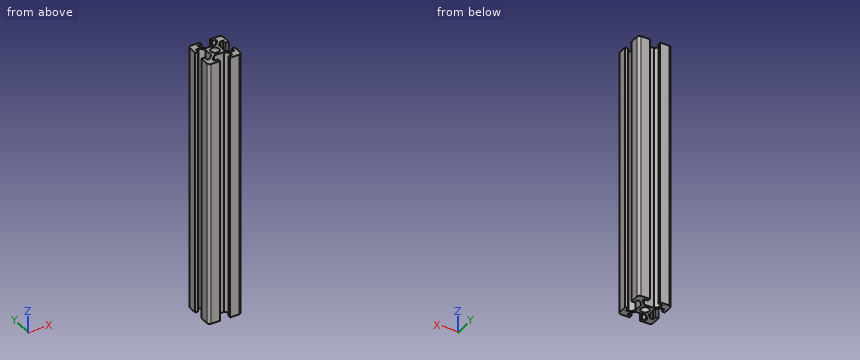
from build123d import *

# Parameters (mm, degrees)
SKETCH_1_R      = 2.5
EXTRUDE_2_DEPTH = 160
SCALE1_SCALE    = 2.5


with BuildPart() as part:
    # 草图1 → 凸台-拉伸2 (new body)
    with BuildSketch(Plane.XY):
        with BuildLine():
            Line((5.5, -8.2), (5.5, -6.560660172))
            Line((5.5, -6.560660172), (2.939339828, -4))
            Line((2.939339828, -4), (-2.939339828, -4))
            Line((-2.939339828, -4), (-5.5, -6.560660172))
            Line((-5.5, -6.560660172), (-5.5, -8.2))
            Line((-5.5, -8.2), (-3.1, -8.2))
            Line((-3.1, -8.2), (-3.1, -10))
            Line((-3.1, -10), (-8.5, -10))
            ThreePointArc((-8.5, -10), (-9.560660172, -9.560660172), (-10, -8.5))
            Line((-10, -8.5), (-10, -3.1))
            Line((-10, -3.1), (-8.2, -3.1))
            Line((-8.2, -3.1), (-8.2, -5.5))
            Line((-8.2, -5.5), (-6.560660172, -5.5))
            Line((-6.560660172, -5.5), (-4, -2.939339828))
            Line((-4, -2.939339828), (-4, 2.939339828))
            Line((-4, 2.939339828), (-6.560660172, 5.5))
            Line((-6.560660172, 5.5), (-8.2, 5.5))
            Line((-8.2, 5.5), (-8.2, 3.1))
            Line((-8.2, 3.1), (-10, 3.1))
            Line((-10, 3.1), (-10, 8.5))
            ThreePointArc((-10, 8.5), (-9.560660172, 9.560660172), (-8.5, 10))
            Line((-8.5, 10), (-3.1, 10))
            Line((-3.1, 10), (-3.1, 8.2))
            Line((-3.1, 8.2), (-5.5, 8.2))
            Line((-5.5, 8.2), (-5.5, 6.560660172))
            Line((-5.5, 6.560660172), (-2.939339828, 4))
            Line((-2.939339828, 4), (2.939339828, 4))
            Line((2.939339828, 4), (5.5, 6.560660172))
            Line((5.5, 6.560660172), (5.5, 8.2))
            Line((5.5, 8.2), (3.1, 8.2))
            Line((3.1, 8.2), (3.1, 10))
            Line((3.1, 10), (8.5, 10))
            ThreePointArc((8.5, 10), (9.560660172, 9.560660172), (10, 8.5))
            Line((10, 8.5), (10, 3.1))
            Line((10, 3.1), (8.2, 3.1))
            Line((8.2, 3.1), (8.2, 5.5))
            Line((8.2, 5.5), (6.560660172, 5.5))
            Line((6.560660172, 5.5), (4, 2.939339828))
            Line((4, 2.939339828), (4, -2.939339828))
            Line((4, -2.939339828), (6.560660172, -5.5))
            Line((6.560660172, -5.5), (8.2, -5.5))
            Line((8.2, -5.5), (8.2, -3.1))
            Line((8.2, -3.1), (10, -3.1))
            Line((10, -3.1), (10, -8.5))
            ThreePointArc((10, -8.5), (9.560660172, -9.560660172), (8.5, -10))
            Line((8.5, -10), (3.1, -10))
            Line((3.1, -10), (3.1, -8.2))
            Line((3.1, -8.2), (5.5, -8.2))
        make_face()
        Circle(SKETCH_1_R, mode=Mode.SUBTRACT)
    extrude(amount=-EXTRUDE_2_DEPTH)


with BuildPart() as part_1:
    # Scale1: scaled about (0, 0, 0)
    add(part.part.scale(SCALE1_SCALE))


solid = part_1.part
Input: part model. Units: mm. Frame: model coordinates. Coordinates: 2 decimals unless noted, no trailing zeros. Loops run counter-clockwise (first coordinate to the right, second up) from the corner with the lowest first, then second, coordinate; pieces in that order, holes last. Notation, with made-up numbers: (74, 66.25) - (104, 66.25) arc R26 cw to (104, 88.25) - close; hole circle Ø10 at (-36, 86.25). An arc over 180 degrees is marked (long way). Answer in a Markdown table with one row per item. Add a question column.
Item 1: Line query: line 1 along X through (y, z) = (13.5, -190); line 2 along X through (y, z) = (8, -186); line 3 along X through (y, z) = (-9.5, -93). Output: solid intervals per line, ascending. Write a range as [from, to].
Item 2: Contact query for flat-ended pins moving along their axis: P1, Ø2, axis at x = 23.5, z = -227.5, coming from the +Y side; P2, Ø12, axis at y = -1.5, z = -172, coming from the +X side; P3, Ø1.3, axis at x = -22.5, z = -266, coming from the +Y side. Output: stop coordinate, or through.
Item 3: Section query A-A on x = 0. Return the cut outline in (y, z).
Recorded:
| question | item | result |
|---|---|---|
| 1 | line 1 | [-25, -20.5], [-16.15, -10.85], [10.85, 16.15], [20.5, 25] |
| 1 | line 2 | [-25, -20.5], [-10.65, 10.65], [20.5, 25] |
| 1 | line 3 | [-25, -20.5], [-12.15, 12.15], [20.5, 25] |
| 2 | P1 | y = 24.79 |
| 2 | P2 | x = 10.15 |
| 2 | P3 | y = 24.95 |
| 3 | outline | (-10, -400) - (-6.25, -400) - (-6.25, 0) - (-10, 0) - close; (6.25, -400) - (10, -400) - (10, 0) - (6.25, 0) - close |
